from build123d import *

# Parameters (mm, degrees)
F0_R      = 92.25
F1_DEPTH  = 114
F2_R      = 92.25
F2_R_2    = 49
F3_DEPTH  = 18
F4_R      = 5
F5_R      = 24
F6_DEPTH  = 26.5
F7_R      = 28.575
F8_DEPTH  = 19
F9_R      = 30
F10_DEPTH = 7.5
F11_R     = 92.25
F11_R_2   = 46
F12_DEPTH = 76
F13_R     = 46
F13_R_2   = 42.5
F14_DEPTH = 12
F15_R     = 31.5
F16_DEPTH = 42
F17_R     = 36.5125
F18_DEPTH = 32.5
F19_R     = 36
F20_DEPTH = 45.5
F21_R     = 11.99999
F22_R     = 5
F23_R     = 92.75
F23_R_2   = 58.66
F24_DEPTH = 23


# Not quite as in the source:
# - a fillet or chamfer is up to 0.001 mm smaller than in the source, because OpenCascade refuses the exact size


with BuildPart() as f1:
    # F0 (on Front) → F1 (new body)
    with BuildSketch(Plane.XZ):
        Circle(F0_R)
    extrude(amount=F1_DEPTH)

    # F2 (on face) → F3 (cut)
    with BuildSketch(Plane.XZ.offset(114)):
        Circle(F2_R)
        Circle(F2_R_2, mode=Mode.SUBTRACT)
    extrude(amount=-F3_DEPTH, mode=Mode.SUBTRACT)

    # F4
    f4_edges = [f1.edges().sort_by_distance(p)[0] for p in [
        (-49, -96, 0),
    ]]
    fillet(f4_edges, radius=F4_R)

    # F5 (on face) → F6 (cut)
    with BuildSketch(Plane.XZ.offset(114)):
        Circle(F5_R)
    extrude(amount=-F6_DEPTH, mode=Mode.SUBTRACT)

    # F7 (on face) → F8 (cut)
    with BuildSketch(Plane.XZ.offset(114)):
        Circle(F7_R)
    extrude(amount=-F8_DEPTH, mode=Mode.SUBTRACT)

    # F9 (on face) → F10 (cut)
    with BuildSketch(Plane.XZ.offset(114)):
        Circle(F9_R)
    extrude(amount=-F10_DEPTH, mode=Mode.SUBTRACT)

    # F11 (on face) → F12 (cut)
    with BuildSketch(Plane(origin=(0, 0, 0), x_dir=(-1, 0, 0), z_dir=(0, 1, 0))):
        Circle(F11_R)
        Circle(F11_R_2, mode=Mode.SUBTRACT)
    extrude(amount=-F12_DEPTH, mode=Mode.SUBTRACT)

    # F13 (on face) → F14 (cut)
    with BuildSketch(Plane(origin=(0, 0, 0), x_dir=(-1, 0, 0), z_dir=(0, 1, 0))):
        Circle(F13_R)
        Circle(F13_R_2, mode=Mode.SUBTRACT)
    extrude(amount=-F14_DEPTH, mode=Mode.SUBTRACT)

    # F15 (on face) → F16 (cut)
    with BuildSketch(Plane(origin=(0, 0, 0), x_dir=(-1, 0, 0), z_dir=(0, 1, 0))):
        Circle(F15_R)
    extrude(amount=-F16_DEPTH, mode=Mode.SUBTRACT)

    # F17 (on face) → F18 (cut)
    with BuildSketch(Plane(origin=(0, 0, 0), x_dir=(-1, 0, 0), z_dir=(0, 1, 0))):
        Circle(F17_R)
    extrude(amount=-F18_DEPTH, mode=Mode.SUBTRACT)

    # F19 (on face) → F20 (cut)
    with BuildSketch(Plane(origin=(0, -42, 0), x_dir=(-1, 0, 0), z_dir=(0, 1, 0))):
        Circle(F19_R)
    extrude(amount=-F20_DEPTH, mode=Mode.SUBTRACT)

    # F21 (radius 12 in the source; OpenCascade refuses exactly that, so slightly less here)
    f21_edges = [f1.edges().sort_by_distance(p)[0] for p in [
        (36, -87.5, 0),
    ]]
    fillet(f21_edges, radius=F21_R)

    # F22
    f22_edges = [f1.edges().sort_by_distance(p)[0] for p in [
        (46, -76, 0),
    ]]
    fillet(f22_edges, radius=F22_R)

    # F23 (on face) → F24 (cut)
    with BuildSketch(Plane.XZ.offset(114)):
        Circle(F23_R)
        Circle(F23_R_2, mode=Mode.SUBTRACT)
    extrude(amount=-F24_DEPTH, mode=Mode.SUBTRACT)


solid = f1.part
Geometry: final body of the model. Coordinates: model frame, mm. A direction names the side the tool comes from. Give positions to 0.01 mm unless a question says otherwise; leave off trailing zeros. Order: outer loops, then holes, each group sorted by start corner. A loop starts at its lowest first (then second) coordinate and runs counter-clockwise, first axis right, second up. Notation, with made-up numbers: (24.5, 33.25) -> (59.5, 33.25) arc R19 ccw to (59.5, 45.25) -> close; hole circle Ø7 at (70, -8.75). An arc over 180 degrees is marked (long way). Put each result on its own line as item: value.
Q1. Draft query along X for faces 4 (the face through (11, -106.5, -27)), 5 (the face through (26, -96, -48)), 6 (the face through (-46.551, -93.535, -35.694)). Return one class per face: released by +X, released by -X, zero draft, split by the parting line, or undercut.
Here are the results:
face 4: undercut
face 5: zero draft
face 6: split by the parting line
Q2. Material intervals for L1, parallel to Z at x = 0, y = -65; L2, parallel to Y at x = 38.5, z = 79.5; L3, parallel to Z at x = 22.5, y = -72.5, sorted ascending.
Here are the results:
L1: z = -46 to -36, 36 to 46
L2: y = -91 to -76
L3: z = -40.39 to -28.1, 28.1 to 40.39
Q3. Reachability of faces 1 (the face through (0, -42, -32)), 2 (the face through (-6.5, -95, 23.4)), 3 (the face through (30, -32.5, -11)) from +Z, -Z, +X, -X, +Y, -Y: full face, straight path, thin tool, end or side. Return the list, or none.
Here are the results:
face 1: none
face 2: -Y
face 3: +Y
Q4. Section A-A, the plane y = -35. Return loops of the section in (x, z), then the cut area to 3 significant figures.
Here are the results:
outline: circle Ø92 at (0, 0); hole circle Ø63 at (0, 0)
area: 3,530 mm^2
Q5. Section B-B, the plane y = -7.5. Return loops of the section in (x, z) (1 decimal), then the cut area to 3 significant figures.
Here are the results:
outline: circle Ø85 at (0, 0); hole circle Ø73 at (0, 0)
area: 1,490 mm^2
Q6. Pin query (flat end, axial travel): pin 1 (4 mm diameter, centred on x = -72.5, z = -56, fed in from -Y); pin 2 (3 mm diameter, centred on x = 24, z = 3.5, fed in from +Y); pin 3 (8 mm diameter, centred on y = -35.5, z = 38, fed in from -X). Return the tip coordinate at first contact, or that it passes through.
Here are the results:
pin 1: stops at y = -91
pin 2: stops at y = -87.37
pin 3: stops at x = -30.98
